Geometry check sheet. Reference: the model listing, model coordinates, mm. A direction names the side the tool comes from. Give positions to 0.01 mm unless a question says otherwise; leave off trailing zeros. Order: outer loops, then holes, each group sorted by start corner. A loop starts at its lowest first (then second) coordinate and runs counter-clockwise, first axis right, second up.
from build123d import *

# Parameters (mm, degrees)
F3_W     = 127
F3_H     = 127
F4_DEPTH = 6.35
F5_DEPTH = 12.7
F0_W     = 63.5
F0_H     = 63.5
F6_DEPTH = 12.7


with BuildPart() as f4:
    # F3 (on Right) → F4 (new body, symmetric)
    with BuildSketch(Plane.YZ):
        with Locations((-63.5, 0)):
            Rectangle(F3_W, F3_H)
    extrude(amount=F4_DEPTH, both=True)

    # F2 (on offset) → F5 (join)
    with BuildSketch(Plane.XZ.offset(127)):
        with BuildLine():
            ThreePointArc((-63.5, 0), (-44.901281, -44.901281), (0, -63.5))
            Line((0, -63.5), (0, 0))
            Line((0, 0), (-63.5, 0))
        make_face()
        with BuildLine():
            ThreePointArc((0, -63.5), (44.901281, -44.901281), (63.5, 0))
            Line((63.5, 0), (0, 0))
            Line((0, 0), (0, -63.5))
        make_face()
        with BuildLine():
            Line((0, 0), (0, 63.5))
            ThreePointArc((0, 63.5), (-44.901281, 44.901281), (-63.5, 0))
            Line((-63.5, 0), (0, 0))
        make_face()
        with BuildLine():
            Line((0, 0), (63.5, 0))
            ThreePointArc((63.5, 0), (44.901281, 44.901281), (0, 63.5))
            Line((0, 63.5), (0, 0))
        make_face()
    extrude(amount=F5_DEPTH)

    # F0 (on Front) → F6 (join)
    with BuildSketch(Plane.XZ):
        with Locations((-31.75, 31.75)):
            Rectangle(F0_W, F0_H)
        with Locations((31.75, 31.75)):
            Rectangle(F0_W, F0_H)
        with Locations((31.75, -31.75)):
            Rectangle(F0_W, F0_H)
        with Locations((-31.75, -31.75)):
            Rectangle(F0_W, F0_H)
    extrude(amount=F6_DEPTH)


solid = f4.part
Item 1: Draft check along Y on faces 4 (the flat face through (-1, 0, 1)), 5 (the flat face through (-35, -12.7, 1)), 6 (the flat face through (-63.5, -6, 1)). Enter one of: released by +Y, released by -Y, zero draft, split by the parting line, or undercut.
Reported:
face 4: released by +Y
face 5: undercut
face 6: zero draft
Item 2: Sectioned sample at D-D (y = -115.5). Enter the section's corners in (x, z).
Reported:
outline: (-6.35, -63.5) - (6.35, -63.5) - (6.35, 63.5) - (-6.35, 63.5) - close
Item 3: Scan lines: L1, parallel to Y at x = 20, z = 53.5; L2, parallel to Y at x = -47, z = 55.5; L3, parallel to X at y = -103.5, z = 35.5. Record each from-to range of solid material in increasing order.
Reported:
L1: y = -139.7 to -127, -12.7 to 0
L2: y = -12.7 to 0
L3: x = -6.35 to 6.35
Item 4: Set-up check for faces 1 (the flat face through (6.35, -71, 1)), 2 (the flat face through (-6.35, -71, 1)), 3 (the flat face through (0, -40, -63.5)): record each of +Z, -Z, +X, -X, +Y, -Y from which the full face is reachable in a straight line by a thin tool's end or side.
Reported:
face 1: +Z, -Z, +X
face 2: +Z, -Z, -X
face 3: -Z, +X, -X, +Y, -Y
Item 5: Gauge pin test, flat ends, axial feed: pin 1 (3 mm diameter, centred on y = -46.5, z = -26.5, fed in from +X); pin 2 (3 mm diameter, centred on y = -50, z = -18.5, fed in from -X). Record the tip position at first contact, or that the pin passes through.
Reported:
pin 1: stops at x = 6.35
pin 2: stops at x = -6.35
Item 6: Sectioned sample at B-B (z = 4). Enter the section's corners in (x, y), and give its area (3 significant figures).
Reported:
outline: (-63.5, -12.7) - (-6.35, -12.7) - (-6.35, -127) - (-63.37, -127) - (-63.37, -139.7) - (63.37, -139.7) - (63.37, -127) - (6.35, -127) - (6.35, -12.7) - (63.5, -12.7) - (63.5, 0) - (-63.5, 0) - close
area: 4,670 mm2
Item 7: Sectioned sample at C-C (x = -34). Enter the section's corners in (y, z), and give its area (3 significant figures).
Reported:
outline: (-139.7, -53.63) - (-127, -53.63) - (-127, 53.63) - (-139.7, 53.63) - close; (-12.7, -63.5) - (0, -63.5) - (0, 63.5) - (-12.7, 63.5) - close
area: 2,980 mm2
Item 8: Sectioned sample at A-A (x = 9.5). Enter the section's corners in (y, z).
Reported:
outline: (-139.7, -62.79) - (-127, -62.79) - (-127, 62.79) - (-139.7, 62.79) - close; (-12.7, -63.5) - (0, -63.5) - (0, 63.5) - (-12.7, 63.5) - close
